Autodesk Inventor part; units mm, degrees
ref_plane "YZ Plane" through (0, 0, 0) normal (1, 0, 0) x (0, 1, 0)
ref_plane "XZ Plane" through (0, 0, 0) normal (0, 1, 0) x (-1, 0, 0)
ref_plane "XY Plane" through (0, 0, 0) normal (0, 0, 1) x (1, 0, 0)
sketch "Sketch1" plane through (0, 0, 0) normal (0, 1, 0) x (-1, 0, 0)
  line L0 (-22, 17.5) -> (22, 17.5)
  line L1 (22, 17.5) -> (22, -17.5)
  line L2 (22, -17.5) -> (-22, -17.5)
  line L3 (-22, -17.5) -> (-22, 17.5)
  line L4 (-22, 17.5) -> (22, -17.5) construction
  line L5 (22, 17.5) -> (-22, -17.5) construction
  point P0 (0, 0)
  dimension "d0" = 44
  dimension "d1" = 35
extrude "Extrusion1" add sketch "Sketch1" along normal mid plane 22
sketch "Sketch2" plane through (-22, 11, 17.5) normal (0, 0, 1) x (1, 0, 0)
  line L0 (3, -0.5) -> (44, -0.5)
  line L1 (44, -0.5) -> (44, -21.5)
  line L2 (44, -21.5) -> (3, -21.5)
  line L3 (3, -21.5) -> (3, -0.5)
  line L4 (0, 0) -> (0, -22)
  line L5 (44, 0) -> (0, 0)
  line L6 (0, -22) -> (44, -22)
  line L7 (44, 0) -> (44, -22)
  point P0 (22, -11)
  dimension "d4" = 3
  dimension "d5" = 0.5
  dimension "d6" = 0.5
  dimension "d7" = 0
extrude "Extrusion2" add sketch "Sketch2" along normal blind 3 contours L0 L1 L2 L3
fillet "Fillet1" radius 10.5 1 edges at (22, 10.5, 19)
fillet "Fillet2" radius 10.5 1 edges at (22, -10.5, 19)
sketch "Sketch3" plane through (-22, 11, 20.5) normal (0, 0, 1) x (1, 0, 0)
  circle A0 centre (33.5, -11) radius 8.5
  arc A1 (33.5, -21.5) -> (33.5, -0.5) centre (33.5, -11) ccw
  point P0 (22, -11)
  dimension "d13" = 2
extrude "Extrusion3" add sketch "Sketch3" along normal blind 1
sketch "Sketch4" plane through (11.5, 0, 21.5) normal (0, 0, 1) x (1, 0, 0)
  circle A0 centre (0, 0) radius 5.5
  circle A1 centre (0, 0) radius 8.5
  point P0 (-11.5, 0)
  dimension "d16" = 3
extrude "Extrusion4" add sketch "Sketch4" along normal blind 3 contours A0
sketch "Sketch5" plane through (11.5, 0, 24.5) normal (0, 0, 1) x (1, 0, 0)
  circle A0 centre (0, 0) radius 13
  point P0 (-11.5, 0)
  dimension "d19" = 26
extrude "Extrusion5" add sketch "Sketch5" along normal blind 1.5
sketch "Sketch7" plane through (-22, -11, 17.5) normal (-1, 0, 0) x (0, 0, 1)
  line L0 (-4, 22) -> (-7, 22)
  line L1 (-7, 22) -> (-7, 0)
  line L2 (-7, 0) -> (-4, 0)
  line L3 (-4, 0) -> (-4, 22)
  line L4 (0, 22) -> (0, 0)
  line L5 (-35, 22) -> (0, 22)
  line L6 (-35, 0) -> (0, 0)
  point P0 (-17.5, 11)
  dimension "d22" = 4
  dimension "d23" = 3
  dimension "d24" = 0
  dimension "d25" = 0
extrude "Extrusion6" add sketch "Sketch7" along normal blind 6 contours L3 L2 L1 L0
sketch "Sketch8" plane through (-22, -11, 13.5) normal (0, 0, 1) x (1, 0, 0)
  circle A0 centre (-4.3, 16) radius 3.5
  circle A1 centre (-4.3, 6) radius 3.5
  line L0 (0, 0) -> (-6, 0)
  line L1 (0, 22) -> (-6, 22)
  line L2 (-6, 0) -> (-6, 22)
  point P0 (22, 11)
  dimension "d28" = 7
  dimension "d29" = 6
  dimension "d30" = 7
  dimension "d31" = 6
  dimension "d32" = 1.7
  dimension "d33" = 1.7
extrude "Extrusion7" cut sketch "Sketch8" against normal through all
mirror "Mirror1" about plane through (0, 0, 0) normal (1, 0, 0) of "Extrusion6", "Extrusion7"
properties part number "servo"
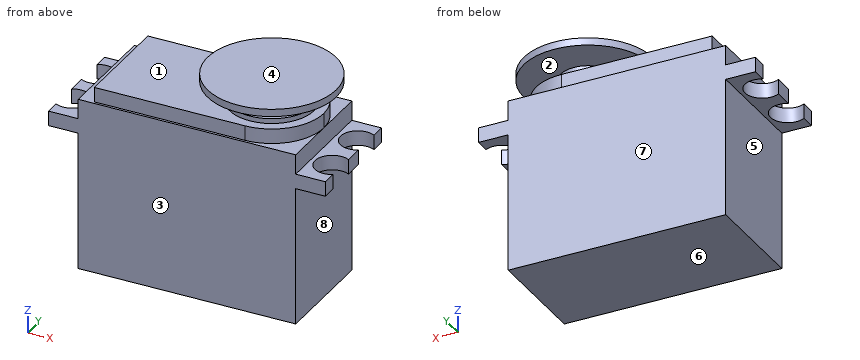
Work out the finished part from the listing and answer in its coordinate system (mm). Face numbers are marked on the shaded views. A direction names the side the tool comes from. Round coordinates to 2 decimals unless told otherwise and drop trailing zeros. Order: outer loops, then holes, each group sorted by start corner. A loop starts at its lowest first (then second) coordinate and runs counter-clockwise, first axis right, second up.
Q1. A cutting plane is placed at D-D, the plane z = 3. Determine the outline of the cut face in (x, y).
Solution:
outline: (-22, -11) - (22, -11) - (22, 11) - (-22, 11) - close
Q2. A cutting plane is placed at A-A, the plane x = 26.3. Determine the outline of the cut face in (y, z).
Solution:
outline: (-11, 10.5) - (-8.5, 10.5) - (-8.5, 13.5) - (-11, 13.5) - close; (-1.5, 10.5) - (1.5, 10.5) - (1.5, 13.5) - (-1.5, 13.5) - close; (8.5, 10.5) - (11, 10.5) - (11, 13.5) - (8.5, 13.5) - close
Q3. A tool of negligible diameter and unlimited length cuts with its end or side. For the marked faces 5, 6, 7 and 8, from which of +Z, -Z, +X, -X, +Y, -Y can it reach the whole face along a straight path? Write none if from no direction.
Solution:
face 5: -Z, -X, +Y, -Y
face 6: -Z, +X, -X, +Y, -Y
face 7: -Z, +X, -X, +Y
face 8: -Z, +X, +Y, -Y
Q4. Find the intervals of material crossed by line 1 along Y through (x, z) = (26, 12); line 2 along Z through (x, y) = (13.5, -9.75); line 3 along Z through (x, y) = (-17, 8.75), in increasing order.
Solution:
line 1: y = -11 to -8.49, -1.51 to 1.51, 8.49 to 11
line 2: z = -17.5 to 20.5, 24.5 to 26
line 3: z = -17.5 to 20.5
Q5. A cutting plane is placed at C-C, the plane y = 4. Determine the outline of the cut face in (x, z), then the cut area to 3 significant figures.
Solution:
outline: (-22.95, 10.5) - (-22, 10.5) - (-22, -17.5) - (22, -17.5) - (22, 10.5) - (22.95, 10.5) - (22.95, 13.5) - (22, 13.5) - (22, 17.5) - (21.21, 17.5) - (21.21, 20.5) - (19, 20.5) - (19, 21.5) - (15.27, 21.5) - (15.27, 24.5) - (23.87, 24.5) - (23.87, 26) - (-0.87, 26) - (-0.87, 24.5) - (7.73, 24.5) - (7.73, 21.5) - (4, 21.5) - (4, 20.5) - (-19, 20.5) - (-19, 17.5) - (-22, 17.5) - (-22, 13.5) - (-22.95, 13.5) - close
area: 1,740 mm2
Q6. Given pin 1 Ø1.5 at (x, z) = (-7.5, 19.5) entering from -Y; pin 2 Ø10 at (x, z) = (5.5, 10.5) entering from -Y; pin 3 Ø4.5 at (y, z) = (-3.5, 16) entering from -X; pin 4 Ø5.5 at (x, y) = (-26.3, -5) entering from -Z, each flat-ended and moving along its own axis, determine where each tip first touches the part or whether it passes through.
Solution:
pin 1: stops at y = -10.5
pin 2: stops at y = -11
pin 3: stops at x = -22
pin 4: passes through
Q7. The mould has two halves that part along Z. Classify the marked faces 1, 2, 3 and 4: pulls with the +Z half, pulls with the -Z half, needs draft (parallel to the pull), parting line crosses it, or undercut.
Solution:
face 1: undercut
face 2: undercut
face 3: needs draft
face 4: pulls with the +Z half
Q8. A cutting plane is placed at B-B, the plane x = 1. Determine the outline of the cut face in (y, z), then the cut area to 3 significant figures.
Solution:
outline: (-11, -17.5) - (11, -17.5) - (11, 17.5) - (10.5, 17.5) - (10.5, 20.5) - (-10.5, 20.5) - (-10.5, 17.5) - (-11, 17.5) - close; (-7.66, 24.5) - (7.66, 24.5) - (7.66, 26) - (-7.66, 26) - close
area: 856 mm2
